Autodesk Fusion 360 part; units mm, degrees
sketch "Skizze1" plane through (0, 0, 0) normal (0, 0, 1) x (1, 0, 0)
  line L0 (-75, 50) -> (-47.27, 50)
  line L1 (-47.27, 50) -> (-47.27, 35.3603)
  line L2 (-47.27, 35.3603) -> (-75, 35.3603)
  line L3 (-75, 35.3603) -> (-75, 50)
  line L4 (-69.4, 50) -> (-69.4, 35.3603)
  line L5 (-66.5, 50) -> (-66.5, 35.3603)
  dimension "d1" = 27.73
  dimension "d2" = 5.6
  dimension "d3" = 2.9
extrude "Extrusion1" add sketch "Skizze1" along normal blind 2.7 contours L0 L2 L3 L4 | L0 L1 L2 L5 makes body 1 at (-73.1333, 45.1201, 0) makes body 2 at (-60.09, 45.1201, 0)
extrude "Extrusion2" add sketch "Skizze1" along normal blind 36.7 contours L0 L2 L4 L5 bodies 1 2
sketch "Skizze2" plane through (-69.4, 0, 0) normal (-1, 0, 0) x (0, -1, 0)
  line L0 (-50, 2.7) -> (-35.3603, 2.7)
  line L1 (-35.3603, 2.7) -> (-35.3603, 36.7)
  line L2 (-35.3603, 36.7) -> (-50, 36.7)
  line L3 (-50, 36.7) -> (-50, 2.7)
  line L4 (-42.6802, 2.7) -> (-42.6802, 36.7) construction
  line L5 (-50, 12.7) -> (-35.3603, 12.7) construction
  line L6 (-50, 2.7) -> (-35.3603, 2.7) construction
  circle A0 centre (-42.6802, 12.7) radius 3.15
  dimension "d8" = 10
  dimension "d9" = 6.3
extrude "Extrusion3" cut sketch "Skizze2" against normal blind 3 contours A0 bodies 1
fillet "Abrundung1" radius 5.5 2 edges at (-75, 50, 1.35) (-75, 35.3603, 1.35) on bodies 1
sketch "Skizze3" plane through (0, 0, 2.7) normal (0, 0, 1) x (-1, 0, 0)
  line L0 (47.27, -50) -> (66.5, -50)
  line L1 (66.5, -50) -> (66.5, -35.3603)
  line L2 (66.5, -35.3603) -> (47.27, -35.3603)
  line L3 (47.27, -35.3603) -> (47.27, -50)
  line L4 (66.5, -38.1003) -> (47.27, -38.1003)
  line L5 (47.27, -47.26) -> (66.5, -47.26)
  line L6 (57.5, -38.1003) -> (57.5, -35.3603)
  line L7 (57.5, -47.26) -> (57.5, -50)
  dimension "d14" = 2.74
  dimension "d15" = 2.74
  dimension "d16" = 9
  dimension "d17" = 9
extrude "Extrusion4" add sketch "Skizze3" along normal blind 9 contours L0 L1 L5 L7 | L1 L2 L4 L6 bodies 1
chamfer "Fase2" distance 9 angle 45 2 edges at (-57.5, 36.7303, 11.7) (-57.5, 48.63, 11.7) on bodies 1
fillet "Abrundung2" radius 1 2 edges at (-69.4, 50, 19.7) (-69.4, 35.3603, 19.7) on bodies 1
fillet "Abrundung3" radius 2 2 edges at (-47.27, 50, 1.35) (-47.27, 35.3603, 1.35) on bodies 1
equation "d1 = 20 mm + 7.73 mm"
equation "d6 = 34 mm + 2.7 mm"
equation "d18 = 15 mm - 2.7 mm - 3.3 mm"
Geometry check sheet. Reference: the model listing, model coordinates, mm. A direction names the side the tool comes from. Coordinates: 2 decimals unless noted, no trailing zeros. Write each loop counter-clockwise with the first axis right and the second up, starting at its lowest first coordinate (ties: lowest second). Pieces come first, ordered by that corner, then holes. Notation, with made-up numbers: (19, 43) -> (24, 43) arc R20 cw to (24, 48) -> close; hole circle Ø11 at (-15, 21). An arc over 180 degrees is marked (long way). One line per question, with ' | ' between items.
1. Draft check along Y on faces 4 (the flat face through (-63.9, 50, 8.7)), 5 (the cylindrical face through (-67.97, 39.77, 11.49)), 6 (the flat face through (-68, 43, 36.7)). Enter one of: +Y half, -Y half, draft (parallel to the pull), parting line (faces both ways), or undercut.
Answers:
face 4: +Y half | face 5: undercut | face 6: draft
2. Cross-section at A-A on z = 12.7. Record the cut outline in (x, y).
Answers:
outline: (-69.4, 36.36) arc R1 ccw to (-68.4, 35.36) -> (-66.5, 35.36) -> (-66.5, 39.53) -> (-69.4, 39.53) -> close; (-69.4, 45.83) -> (-66.5, 45.83) -> (-66.5, 50) -> (-68.4, 50) arc R1 ccw to (-69.4, 49) -> close
3. Cross-section at B-B on y = 42. Record the cut outline in (x, z), and give its area (3 significant figures).
Answers:
outline: (-75, 0) -> (-47.27, 0) -> (-47.27, 2.7) -> (-66.5, 2.7) -> (-66.5, 9.62) -> (-69.4, 9.62) -> (-69.4, 2.7) -> (-75, 2.7) -> close; (-69.4, 15.78) -> (-66.5, 15.78) -> (-66.5, 36.7) -> (-69.4, 36.7) -> close | area: 156 mm²
4. Cross-section at C-C on x = -69. Record the cut outline in (y, z), and give its area (3 significant figures).
Answers:
outline: (35.36, 0) -> (50, 0) -> (50, 2.7) -> (49.8, 2.7) -> (49.8, 36.7) -> (35.56, 36.7) -> (35.56, 2.7) -> (35.36, 2.7) -> close; hole circle Ø6.3 at (42.68, 12.7) | area: 493 mm²
5. Cross-section at D-D on y = 39. Record the cut outline in (x, z), and give its area (3 significant figures).
Answers:
outline: (-74.68, 0) -> (-47.27, 0) -> (-47.27, 2.7) -> (-66.5, 2.7) -> (-66.5, 36.7) -> (-69.4, 36.7) -> (-69.4, 2.7) -> (-74.68, 2.7) -> close | area: 173 mm²
6. Set-up check for faces 1 (the cylindrical face through (-69.115, 35.661, 19.938)), 2 (the cylindrical face through (-69.099, 49.715, 19.938)), 3 (the flat face through (-63, 47.26, 6)): record each of +Z, -Z, +X, -X, +Y, -Y from which the full face is reachable in a straight line by a thin tool's end or side.
Answers:
face 1: +Z, -X, -Y | face 2: +Z, -X, +Y | face 3: +Z, +X
7. Depth check by flat-ended pin: pin 1 Ø2 at (y, z) = (44, 4.5) entering from +X; pin 2 Ø4.5 at (x, y) = (-55, 44.5) entering from +Z; pin 3 Ø1.5 at (x, z) = (-64.5, 22.5) entering from -Y. Enter the tip coordinate at first touch or a pass-through.
Answers:
pin 1: stops at x = -66.5 | pin 2: stops at z = 2.7 | pin 3: passes through
8. Thickness scan on probe 1 along X at (y, z) = (47.75, 18.5); probe 2 along Z at (x, y) = (-49.5, 45.75); probe 3 along Z at (x, y) = (-62, 37.5). Record the ranges inside material, lowest first. Write a range as from..to.
Answers:
probe 1: x = -69.4..-66.5 | probe 2: z = 0..2.7 | probe 3: z = 0..7.2
